Input: part model. Units: mm. Frame: model coordinates. Face numbers are marked on the shaded views. A direction names the side the tool comes from. Coordinates: 2 decimals unless noted, no trailing zeros. Order: outer loops, then holes, each group sorted by start corner. A loop starts at its lowest first (then second) coordinate and runs counter-clockwise, first axis right, second up. Notation, with made-up numbers: (4, 45) -> (40, 45) arc R32 ccw to (40, 73) -> close; hole circle Ø6 at (85, 21.5). An arc over 180 degrees is marked (long way). Use CSV: the item, a comma, the result in double quotes. Start each with the question number.
```python
from build123d import *

# Parameters (mm, degrees)
F2_W     = 700
F2_H     = 242
F2_W_2   = 220
F2_H_2   = 106
F3_DEPTH = 86
F4_DEPTH = 76


with BuildPart() as f3:
    # F2 (on Top) → F3 (new body)
    with BuildSketch(Plane.XY):
        with Locations((79.4747328101, 7.7042136107)):
            Rectangle(F2_W, F2_H)
        with Locations((-150.5252671899, -50.2957863893)):
            Rectangle(F2_W_2, F2_H_2, mode=Mode.SUBTRACT)
        with Locations((79.4747328101, -50.2957863893)):
            Rectangle(F2_W_2, F2_H_2, mode=Mode.SUBTRACT)
        with Locations((309.4747328101, -50.2957863893)):
            Rectangle(F2_W_2, F2_H_2, mode=Mode.SUBTRACT)
        with Locations((-150.5252671899, 65.7042136107)):
            Rectangle(F2_W_2, F2_H_2, mode=Mode.SUBTRACT)
        with Locations((79.4747328101, 65.7042136107)):
            Rectangle(F2_W_2, F2_H_2, mode=Mode.SUBTRACT)
        with Locations((309.4747328101, 65.7042136107)):
            Rectangle(F2_W_2, F2_H_2, mode=Mode.SUBTRACT)
        with Locations((-150.5252671899, 65.7042136107)):
            Rectangle(F2_W_2, F2_H_2)
        with Locations((-150.5252671899, -50.2957863893)):
            Rectangle(F2_W_2, F2_H_2)
        with Locations((79.4747328101, -50.2957863893)):
            Rectangle(F2_W_2, F2_H_2)
        with Locations((79.4747328101, 65.7042136107)):
            Rectangle(F2_W_2, F2_H_2)
        with Locations((309.4747328101, 65.7042136107)):
            Rectangle(F2_W_2, F2_H_2)
        with Locations((309.4747328101, -50.2957863893)):
            Rectangle(F2_W_2, F2_H_2)
    extrude(amount=-F3_DEPTH)

    # F2 (on Top) → F4 (cut)
    with BuildSketch(Plane.XY):
        with Locations((-150.5252671899, 65.7042136107)):
            Rectangle(F2_W_2, F2_H_2)
        with Locations((-150.5252671899, -50.2957863893)):
            Rectangle(F2_W_2, F2_H_2)
        with Locations((79.4747328101, 65.7042136107)):
            Rectangle(F2_W_2, F2_H_2)
        with Locations((79.4747328101, -50.2957863893)):
            Rectangle(F2_W_2, F2_H_2)
        with Locations((309.4747328101, 65.7042136107)):
            Rectangle(F2_W_2, F2_H_2)
        with Locations((309.4747328101, -50.2957863893)):
            Rectangle(F2_W_2, F2_H_2)
    extrude(amount=-F4_DEPTH, mode=Mode.SUBTRACT)


solid = f3.part
```
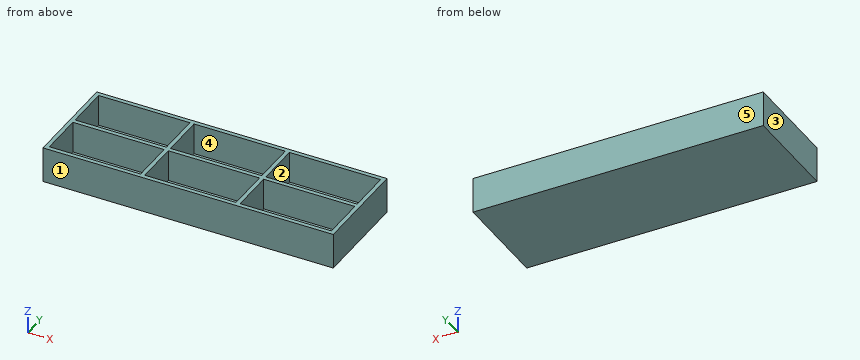
1. Access query for the marked faces 1 and 2. Directions: +Z, -Z, +X, -X, +Y, -Y. A direction counts if a zero-diameter tool reaches every point of the face in a straight line with its end or side. Return the directions, or none.
2. Section A-A on z = -54. Return loops of the section in (x, y), then the cut area to 3 significant figures.
3. Section C-C on y = -38. Return loops of the section in (x, z), then the cut area to 3 significant figures.
4. Section B-B on x = 251. Return loops of the section in (y, z), then the cut area to 3 significant figures.
5. Pull-direction query (Y, two-part tool) for the marked faces 3, 4 and 5; classes: released by +Y, released by -Y, zero draft, split by the parting line, or undercut.
6. Material intervals for line 1 along Y through (x, z) = (158.5, -33); line 2 along X through (y, z) = (-82, -74.5); line 3 along Z through (x, y) = (392, 67), sorted ascending.
7. Contact query for a flat-ended pin moving along its axis: P1, Ø5, axis at x = -87.5, y = 27, coming from the +Z side. Output: stop coordinate, or through.
Values follow:
1,face 1,"+Z, -Z, +X, -X, -Y"
1,face 2,"+Z"
2,outline,"(-270.53, -113.3) -> (429.47, -113.3) -> (429.47, 128.7) -> (-270.53, 128.7) -> close; hole (-260.53, -103.3) -> (-40.53, -103.3) -> (-40.53, 2.7) -> (-260.53, 2.7) -> close; hole (-260.53, 12.7) -> (-40.53, 12.7) -> (-40.53, 118.7) -> (-260.53, 118.7) -> close; hole (-30.53, -103.3) -> (189.47, -103.3) -> (189.47, 2.7) -> (-30.53, 2.7) -> close; hole (-30.53, 12.7) -> (189.47, 12.7) -> (189.47, 118.7) -> (-30.53, 118.7) -> close; hole (199.47, -103.3) -> (419.47, -103.3) -> (419.47, 2.7) -> (199.47, 2.7) -> close; hole (199.47, 12.7) -> (419.47, 12.7) -> (419.47, 118.7) -> (199.47, 118.7) -> close"
2,area,"29,500 mm2"
3,outline,"(-270.53, -86) -> (429.47, -86) -> (429.47, 0) -> (419.47, 0) -> (419.47, -76) -> (199.47, -76) -> (199.47, 0) -> (189.47, 0) -> (189.47, -76) -> (-30.53, -76) -> (-30.53, 0) -> (-40.53, 0) -> (-40.53, -76) -> (-260.53, -76) -> (-260.53, 0) -> (-270.53, 0) -> close"
3,area,"10,000 mm2"
4,outline,"(-113.3, -86) -> (128.7, -86) -> (128.7, 0) -> (118.7, 0) -> (118.7, -76) -> (12.7, -76) -> (12.7, 0) -> (2.7, 0) -> (2.7, -76) -> (-103.3, -76) -> (-103.3, 0) -> (-113.3, 0) -> close"
4,area,"4,700 mm2"
5,face 3,"zero draft"
5,face 4,"undercut"
5,face 5,"released by +Y"
6,line 1,"y = -113.3 to -103.3, 2.7 to 12.7, 118.7 to 128.7"
6,line 2,"x = -270.53 to -260.53, -40.53 to -30.53, 189.47 to 199.47, 419.47 to 429.47"
6,line 3,"z = -86 to -76"
7,P1,"stops at z = -76"
